Check sheet for the modelled part. Datum: model origin and axes. Units: mm. A direction names the side the tool comes from. Give positions to 0.01 mm unless a question says otherwise; leave off trailing zeros. Write each loop counter-clockwise with the first axis right and the second up, starting at its lowest first coordinate (ties: lowest second). Pieces come first, ordered by that corner, then holes. Notation, with made-up numbers: M 42,79.25 L 72,79.25 A7 cw 72,90.25 Z; hole C -23.75,47 d8. An arc over 180 degrees is marked long. Write item = value, one per line. Start each with the question number.
1) Sectioned sample at A-A, the plane z = -40.5. Record the cut outline in (x, y).
2) Gauge pin test, flat ends, axial feed: pin 1 (2 mm diameter, centred on x = -87.5, z = 107.5, fed in from +Y); pin 2 (1.1 mm diameter, centred on x = -88, z = -191.5, fed in from +Y). Record the tip position at first contact, or that the pin passes through.
3) Scan lines: L1, parallel to X at y = 14, z = -37.25; L2, parallel to Z at x = -4.5, y = 3.5; L3, parallel to X at y = 2, z = -90. Record each from-to range of solid material in increasing order.
4) Sectioned sample at B-B, the plane x = 12. Record the cut outline in (y, z), then the cut area to 3 significant figures.
5) Set-up check for faces 1 (the face through (-91.649, 11, -44)), 2 (the face through (32, 9, -51.573)): record each of +Z, -Z, +X, -X, +Y, -Y from which the full face is reachable in a straight line by a thin tool's end or side.
Autodesk Inventor part; units mm, degrees
ref_plane "YZ Plane" through (0, 0, 0) normal (1, 0, 0) x (0, 1, 0)
ref_plane "XZ Plane" through (0, 0, 0) normal (0, 1, 0) x (-1, 0, 0)
ref_plane "XY Plane" through (0, 0, 0) normal (0, 0, 1) x (1, 0, 0)
sketch "Sketch1" plane through (0, 0, 0) normal (0, 1, 0) x (-1, 0, 0)
  line L0 (80.1493, 105.9266) -> (-24.8507, 105.9266) construction
  line L1 (-24.8507, 105.9266) -> (-24.8507, -189.0734) construction
  line L2 (-24.8507, -189.0734) -> (80.1493, -189.0734) construction
  line L3 (80.1493, -189.0734) -> (80.1493, 105.9266) construction
  line L4 (80.1493, 91.9266) -> (83.1493, 91.9266) construction
  line L5 (83.1493, 91.9266) -> (83.1493, 84.3266) construction
  line L6 (83.1493, 84.3266) -> (80.1493, 84.3266) construction
  line L7 (80.1493, 84.3266) -> (80.1493, 91.9266) construction
  point P0 (0, 0)
  dimension "d0" = 295
  dimension "d1" = 105
  dimension "d2" = 7.6
  dimension "d3" = 3
  dimension "d4" = 14
sketch "Sketch2" plane through (0, 0, 0) normal (0, 1, 0) x (-1, 0, 0)
  line L0 (80.1493, -189.0734) -> (80.1493, 105.9266) construction
  line L1 (-24.8507, -189.0734) -> (80.1493, -189.0734) construction
  line L2 (-24.8507, 105.9266) -> (-24.8507, -189.0734) construction
  line L3 (80.1493, 105.9266) -> (-24.8507, 105.9266) construction
  line L4 (90.1493, 109.9266) -> (90.1493, -193.0734)
  line L5 (-34.8507, -193.0734) -> (-34.8507, 109.9266)
  line L6 (90.1493, 109.9266) -> (-34.8507, 109.9266)
  line L7 (90.1493, -193.0734) -> (-34.8507, -193.0734)
  line L8 (91.6493, -194.5734) -> (91.6493, 111.4266)
  line L9 (91.6493, 111.4266) -> (-36.3507, 111.4266)
  line L10 (-36.3507, 111.4266) -> (-36.3507, -194.5734)
  line L11 (-36.3507, -194.5734) -> (91.6493, -194.5734)
  dimension "d71" = 10
  dimension "d72" = 4
  dimension "d73" = 10
  dimension "d74" = 4
  dimension "d75" = 1.5
extrude "Extrusion1" add sketch "Sketch2" against normal blind 1 contours L4 L7 L5 L6
extrude "Extrusion2" add sketch "Sketch2" along normal blind 23 and the other way blind 1
sketch "Sketch5" plane through (-91.6493, -1, 111.4266) normal (-1, 0, 0) x (0, 0, 1)
  circle A0 centre (-246, 19) radius 2.25
  circle A1 centre (-90.8, 19) radius 2.25
  circle A2 centre (-215.2, 19) radius 2.25
  circle A3 centre (-60, 19) radius 2.25
  line L0 (0, 0) -> (0, 24)
  line L1 (-306, 24) -> (0, 24)
  line L2 (-306, 24) -> (-306, 0)
  line L3 (0, 0) -> (-306, 0)
  point P0 (-111.4266, 1)
  dimension "d35" = 4.5
  dimension "d37" = 4.5
  dimension "d39" = 4.5
  dimension "d40" = 0
  dimension "d41" = 30.8
  dimension "d45" = 4.5
  dimension "d46" = 0
  dimension "d47" = 30.8
  dimension "d76" = 60
  dimension "d77" = 60
  dimension "d144" = 5
  dimension "d145" = 5
extrude "Extrusion4" cut sketch "Sketch5" against normal up to surface (1.5 mm away) contours A0 | A1 | A2 | A3
sketch "Sketch7" plane through (-90.1493, 0, -193.0734) normal (1, 0, 0) x (0, 0, -1)
  line L0 (-151.5, 23) -> (-151.5, 0) construction
  line L1 (-141.5, 19) -> (-141.5, 0)
  line L2 (-161.5, 19) -> (-161.5, 0)
  line L3 (-303, 23) -> (0, 23)
  line L4 (-303, 0) -> (0, 0)
  line L5 (0, 23) -> (0, 0)
  line L6 (-161.5, 19) -> (-141.5, 19)
  point P0 (-141.5, 23)
  point P1 (-161.5, 23)
  dimension "d106" = 10
  dimension "d107" = 10
  dimension "d148" = 151.5
  dimension "d149" = 151.5
  dimension "d193" = 19
extrude "Extrusion6" add sketch "Sketch7" along normal blind 6
ref_plane "Work Plane2" through (-27.6493, 0, 109.9266) normal (1, 0, 0) x (0, 0, -1)
ref_plane "Work Plane4" through (-90.1493, 0, -41.5734) normal (0, 0, 1) x (1, 0, 0)
sketch "Sketch16" plane through (-90.1493, 0, -31.5734) normal (0, 0, 1) x (1, 0, 0)
  line L0 (0, 0) -> (0, 19)
  line L1 (0, 19) -> (6, 19)
  point P0 (90.1493, 0)
  point P1 (3.5, 14)
  dimension "d108" = 3.5
  dimension "d194" = 5
hole "Hole3" at (-86.6493, 14, -31.5734) direction (0, 0, -1) diameter 2.6 depth 5 countersink diameter 5 countersink angle 82
sketch "Sketch17" plane through (-86.6493, 14, -36.5734) normal (0, 0, 1) x (1, 0, 0)
  circle A0 centre (0, 0) radius 1.3
  point P0 (86.6493, -14)
hole "Hole4" at (-86.6493, 14, -36.5734) direction (0, 0, -1) diameter 2.6 depth 15 tip angle 118
sketch "Sketch18" plane through (-90.1493, 0, -31.5734) normal (0, 0, 1) x (1, 0, 0)
  line L0 (0, 0) -> (0, 19)
  line L1 (6, 0) -> (0, 0)
  point P0 (90.1493, 0)
  point P1 (3.5, 5)
  point P2 (0, 18)
  point P3 (0, 23)
  dimension "d124" = 3.5
  dimension "d125" = 5
hole "Hole5" at (-86.6493, 5, -31.5734) direction (0, 0, -1) diameter 2.6 depth 5 countersink diameter 5 countersink angle 82
sketch "Sketch19" plane through (-86.6493, 5, -36.5734) normal (0, 0, 1) x (1, 0, 0)
  circle A0 centre (0, 0) radius 1.3
  point P0 (86.6493, -5)
hole "Hole6" at (-86.6493, 5, -36.5734) direction (0, 0, -1) diameter 2.6 depth 15 tip angle 118
mirror "Mirror6" about plane through (-27.6493, 0, 109.9266) normal (1, 0, 0) of "Extrusion6", "Hole3", "Hole5", "Hole4", "Hole6"
sketch "Sketch23" plane through (0, 0, 0) normal (0, 1, 0) x (1, 0, 0)
  line L0 (-90.1493, 193.0734) -> (34.8507, 193.0734)
  line L1 (34.8507, 193.0734) -> (30.8507, 193.0734)
  line L2 (30.8507, 193.0734) -> (30.8507, 189.0734)
  line L3 (30.8507, 189.0734) -> (34.8507, 189.0734)
  line L4 (34.8507, 189.0734) -> (34.8507, 193.0734)
  circle A0 centre (32.8507, 191.0734) radius 1.1
  line L5 (-90.1493, 193.0734) -> (-86.1493, 193.0734)
  line L6 (-86.1493, 193.0734) -> (-86.1493, 189.0734)
  line L7 (-86.1493, 189.0734) -> (-90.1493, 189.0734)
  line L8 (-90.1493, 189.0734) -> (-90.1493, 193.0734)
  circle A1 centre (-88.1493, 191.0734) radius 1.1
  line L9 (34.8507, -109.9687) -> (30.8507, -109.9687)
  line L10 (30.8507, -109.9687) -> (30.8507, -105.9687)
  line L11 (30.8507, -105.9687) -> (34.8507, -105.9687)
  line L12 (34.8507, -105.9687) -> (34.8507, -109.9687)
  circle A2 centre (32.8507, -107.9687) radius 1.1
  line L13 (34.8507, -109.9266) -> (-90.1493, -109.9266)
  line L14 (-90.1493, -109.9266) -> (-86.1493, -109.9266)
  line L15 (-86.1493, -109.9266) -> (-86.1493, -105.9266)
  line L16 (-86.1493, -105.9266) -> (-90.1493, -105.9266)
  line L17 (-90.1493, -105.9266) -> (-90.1493, -109.9266)
  circle A3 centre (-88.1493, -107.9266) radius 1.1
  point P0 (0, 0)
  dimension "d159" = 4
  dimension "d160" = 4
  dimension "d161" = 2.2
  dimension "d162" = 2
  dimension "d163" = 2
  dimension "d164" = 4
  dimension "d165" = 4
  dimension "d166" = 2.2
  dimension "d167" = 2
  dimension "d168" = 2
  dimension "d169" = 4
  dimension "d170" = 4
  dimension "d171" = 2.2
  dimension "d172" = 2
  dimension "d173" = 2
  dimension "d174" = 4
  dimension "d175" = 4
  dimension "d176" = 2.2
  dimension "d177" = 2
  dimension "d178" = 2
extrude "Extrusion14" add sketch "Sketch23" along normal blind 19
sketch "Sketch24" plane through (-90.1493, 23, -193.0734) normal (0, 0, 1) x (1, 0, 0)
  line L0 (34, -14) -> (43, -14)
  line L1 (43, -14) -> (43, -19)
  line L2 (43, -19) -> (34, -19)
  line L3 (34, -19) -> (34, -14)
  line L4 (4, -23) -> (121, -23)
  line L5 (4, -23) -> (4, -4)
  line L6 (83, -14) -> (92, -14)
  line L7 (92, -14) -> (92, -19)
  line L8 (92, -19) -> (83, -19)
  line L9 (83, -19) -> (83, -14)
  point P0 (90.1493, -23)
  dimension "d181" = 9
  dimension "d182" = 5
  dimension "d183" = 4
  dimension "d184" = 30
  dimension "d187" = 9
  dimension "d188" = 5
  dimension "d189" = 40
  dimension "d190" = 4
extrude "Extrusion15" cut sketch "Sketch24" against normal through all
sketch "Sketch25" plane through (-90.1493, 0, -41.5734) normal (0, 0, 1) x (1, 0, 0)
  line L0 (169.9232, 195.9359) -> (-46.5393, 195.9359)
  line L1 (-46.5393, 195.9359) -> (-46.5393, -158.6148)
  line L2 (-46.5393, -158.6148) -> (169.9232, -158.6148)
  line L3 (169.9232, -158.6148) -> (169.9232, 195.9359)
  point P0 (90.1493, 0)
extrude "Extrusion16" [suppressed]
sketch "Sketch27" plane through (0, 23, 0) normal (0, 1, 0) x (1, 0, 0)
  line L0 (34.8507, 193.0734) -> (34.8507, -109.9266)
  line L1 (-90.1493, 193.0734) -> (34.8507, 193.0734)
  line L2 (-90.1493, -109.9266) -> (-90.1493, 193.0734)
  line L3 (34.8507, -109.9266) -> (-90.1493, -109.9266)
  line L4 (-90.1493, 136.8234) -> (-90.1493, 132.3234)
  line L5 (-91.6493, 132.3234) -> (-91.6493, 136.8234)
  line L6 (-91.6493, 101.5234) -> (-91.6493, 106.0234)
  line L7 (-91.6493, -22.8766) -> (-91.6493, -18.3766)
  line L8 (-91.6493, -53.6766) -> (-91.6493, -49.1766)
  point P0 (0, 0)
  dimension "d196" = 56.25
  dimension "d197" = 4.5
  dimension "d198" = 26.3
  dimension "d199" = 4.5
  dimension "d200" = 119.9
  dimension "d201" = 4.5
  dimension "d202" = 26.3
  dimension "d203" = 4.5
  dimension "d204" = 56.25
properties part number "Case Board"
Data:
q1.outline = M -91.65,-1 L 36.35,-1 L 36.35,23 L 34.85,23 L 34.85,19 L 28.85,19 L 28.85,0 L -84.15,0 L -84.15,19 L -90.15,19 L -90.15,23 L -91.65,23 Z; hole C -86.65,5 d2.6; hole C -86.65,14 d2.6; hole C 31.35,5 d2.6; hole C 31.35,14 d2.6
q2.pin_1 = 19
q2.pin_2 = 0
q3.L1 = -91.65 to -87.95, -85.35 to -84.15, 28.85 to 30.05, 32.65 to 36.35
q3.L2 = -194.57 to -193.07, 109.93 to 111.43
q3.L3 = -91.65 to -90.15, 34.85 to 36.35
q4.outline = M -1,-194.57 L 23,-194.57 L 23,-193.07 L 0,-193.07 L 0,109.93 L 23,109.93 L 23,111.43 L -1,111.43 Z
q4.area = 375 mm2
q5.face_1 = +Z, -Z, -X, +Y, -Y
q5.face_2 = +Y
